Here's how the part is built. I have some questions about the finished solid (model axes, mm). A direction names the side the tool comes from. Round coordinates to 2 decimals unless told otherwise and drop trailing zeros. Loops run counter-clockwise (first coordinate to the right, second up) from the corner with the lowest first, then second, coordinate; pieces in that order, holes last. Notation, with made-up numbers: (83, 38) -> (138, 38) arc R28 cw to (138, 71) -> close; hole circle Ø8 at (42, 44). An arc over 180 degrees is marked (long way). Use one line per item in the form item = value. Start each with the question number.
Item 1: If we section it at A-A (x = 9): Write out the boundary of the cut face in (y, z).
Item 2: If we section it at D-D (y = 4): Write out the boundary of the cut face in (x, z).
Item 3: For faces 1 (the face through (-2.17, -11.08, -9.76)), 2 (the face through (7.155, -2.465, -5.591)), 3 (the face through (0, -6.4, 0)), which set-ups out of +Z, -Z, +X, -X, +Y, -Y let a thin tool reach every point of the face, with its end or its side?
Item 4: If we section it at C-C (z = -8): Write out the boundary of the cut face in (x, y), then the cut area to 3 significant figures.
Item 5: If we section it at B-B (y = -3.75): State how many separate pieces and enclosed holes the cut face has, then the cut area to 3 significant figures.
Item 6: Thinking about a two-plate mould opening in Z: for faces 4 (the face through (0, -8, 0)), 5 (the face through (4, 0, 0)), 6 (the face through (-2.25, 3.45, 0.71)), which applies, released by +Z, released by -Z, zero draft, split by the parting line, or undercut?
Item 7: If I drill on L1, parallel to Z at x = -2.5, y = -5.5; L2, parallel to Z at x = 8, y = -2; L3, parallel to X at y = -12.5, z = -8.5, over which ranges is the centre line in solid material (lowest first)? Write a range as [from, to].
Item 8: I'm going to push flat-ended pins straight in: pin 1 Ø1 at (x, z) = (0, 0) entering from +Y; pin 2 Ø6 at (y, z) = (1.5, -14.5) entering from +X; pin 3 Ø2 at (x, z) = (0.5, -0.5) entering from -Y; pin 4 Ø2.5 at (x, z) = (0, -8) entering from +Y. Where does each tip first touch, or does it pass through?
```python
from build123d import *

# Parameters (mm, degrees)
F0_R      = 19.5
F1_DEPTH  = 17
F2_R      = 10
F3_DEPTH  = 12
F4_R      = 1.5
F5_DEPTH  = 25
F6_R      = 6.5
F7_DEPTH  = 1
F8_R      = 0.1455076687
F9_DEPTH  = 0.1
F11_R     = 1.3872068032
F12_DEPTH = 2
F13_R     = 2.3581013166
F14_DEPTH = 7
F15_R     = 0.8149743097
F16_DEPTH = 13.4


with BuildPart() as f1:
    # F0 (on Front) → F1 (new body)
    with BuildSketch(Plane.XZ):
        Circle(F0_R)
    extrude(amount=F1_DEPTH)

    # F2 (on face) → F3 (cut)
    with BuildSketch(Plane.XZ.offset(17)):
        Circle(F2_R)
    extrude(amount=-F3_DEPTH, mode=Mode.SUBTRACT)

    # F4 (on face) → F5 (cut)
    with BuildSketch(Plane(origin=(0, 0, 0), x_dir=(-1, 0, 0), z_dir=(0, 1, 0))):
        with BuildLine():
            ThreePointArc((0, 9.5), (-1.5, 8), (0, 6.5))
            ThreePointArc((0, 6.5), (1.0606601718, 6.9393398282), (1.5, 8))
            ThreePointArc((1.5, 8), (1.0606601718, 9.0606601718), (0, 9.5))
        make_face()
        with Locations((-5.6568542495, 5.6568542495)):
            Circle(F4_R)
        with Locations((-8, 0)):
            Circle(F4_R)
        with Locations((-5.6568542495, -5.6568542495)):
            Circle(F4_R)
        with Locations((0, -8)):
            Circle(F4_R)
        with Locations((5.6568542495, -5.6568542495)):
            Circle(F4_R)
        with Locations((8, 0)):
            Circle(F4_R)
        with Locations((5.6568542495, 5.6568542495)):
            Circle(F4_R)
    extrude(amount=-F5_DEPTH, mode=Mode.SUBTRACT)

    # F6 (on face) → F7 (join)
    with BuildSketch(Plane.XZ.offset(5)):
        Circle(F6_R)
        with BuildLine():
            ThreePointArc((4.5961940604, -4.596194095), (6.0052169566, -2.4874423217), (6.5, 0))
            ThreePointArc((6.5, 0), (6.0052169613, 2.4874423104), (4.5961940777, 4.5961940777))
            ThreePointArc((4.5961940777, 4.5961940777), (2.4874423104, 6.0052169613), (0, 6.5))
            ThreePointArc((0, 6.5), (-2.4874423043, 6.0052169639), (-4.5961940684, 4.5961940871))
            ThreePointArc((-4.5961940684, 4.5961940871), (-6.0052169588, 2.4874423165), (-6.5, 0))
            ThreePointArc((-6.5, 0), (-6.0052169618, -2.4874423093), (-4.5961940793, -4.5961940761))
            ThreePointArc((-4.5961940793, -4.5961940761), (-2.4874423124, -6.0052169605), (-2.2e-09, -6.5))
            ThreePointArc((-2.2e-09, -6.5), (2.487442298, -6.0052169664), (4.5961940604, -4.596194095))
        make_face()
    extrude(amount=F7_DEPTH)

    # F8 (on face) → F9 (join)
    with BuildSketch(Plane.XZ.offset(6)):
        with Locations((0, 6.145354826)):
            Circle(F8_R)
        with Locations((-3.6121489368, 4.9716964907)):
            Circle(F8_R)
        with Locations((-5.8445797522, 1.8990190777)):
            Circle(F8_R)
        with Locations((-5.8445797522, -1.8990190777)):
            Circle(F8_R)
        with Locations((-3.6121489368, -4.9716964907)):
            Circle(F8_R)
        with Locations((0, -6.145354826)):
            Circle(F8_R)
        with Locations((3.6121489368, -4.9716964907)):
            Circle(F8_R)
        with Locations((5.8445797522, -1.8990190777)):
            Circle(F8_R)
        with Locations((5.8445797522, 1.8990190777)):
            Circle(F8_R)
        with Locations((3.6121489368, 4.9716964907)):
            Circle(F8_R)
    extrude(amount=F9_DEPTH)

    # F11 (on face) → F12 (join)
    with BuildSketch(Plane.XZ.offset(6)):
        Circle(F11_R)
    extrude(amount=F12_DEPTH)

    # F13 (on face) → F14 (join)
    with BuildSketch(Plane(origin=(0, 0, 0), x_dir=(-1, 0, 0), z_dir=(0, 1, 0))):
        Circle(F13_R)
    extrude(amount=F14_DEPTH)

    # F15 (on face) → F16 (cut)
    with BuildSketch(Plane(origin=(0, 7, 0), x_dir=(-1, 0, 0), z_dir=(0, 1, 0))):
        Circle(F15_R)
    extrude(amount=-F16_DEPTH, mode=Mode.SUBTRACT)


solid = f1.part
```
Values found:
q1.outline = (-17, -17.3) -> (0, -17.3) -> (0, -1.12) -> (-5, -1.12) -> (-5, -4.36) -> (-17, -4.36) -> close; (-17, 4.36) -> (-5, 4.36) -> (-5, 1.12) -> (0, 1.12) -> (0, 17.3) -> (-17, 17.3) -> close
q2.outline = circle Ø4.72 at (0, 0); hole circle Ø1.63 at (0, 0)
q3.face_1 = -Y
q3.face_2 = +Y, -Y
q3.face_3 = +Y
q4.outline = (-17.78, -17) -> (-6, -17) -> (-6, -5) -> (-1.5, -5) -> (-1.5, 0) -> (-17.78, 0) -> close; (1.5, -5) -> (6, -5) -> (6, -17) -> (17.78, -17) -> (17.78, 0) -> (1.5, 0) -> close
q4.area = 446 mm2
q5.separate_pieces = 1
q5.enclosed_holes = 9
q5.area = 1,140 mm2
q6.face_4 = undercut
q6.face_5 = zero draft
q6.face_6 = split by the parting line
q7.L1 = [-19.34, -9.68], [-6, 6], [9.68, 19.34]
q7.L2 = [-17.78, -1.5], [1.5, 17.78]
q7.L3 = [-17.55, -5.27], [5.27, 17.55]
q8.pin_1 = -6.4
q8.pin_2 = 15.45
q8.pin_3 = -8
q8.pin_4 = through
